Build history of the part. All positions in model axes, mm. A direction names the side the tool comes from. Round coordinates to 2 decimals unless told otherwise and drop trailing zeros. Write each loop counter-clockwise with the first axis right and the second up, starting at its lowest first coordinate (ties: lowest second). Pieces come first, ordered by that corner, then holes. Notation, with made-up numbers: M 3,-17 L 43,-17 A21 ccw 43,1 Z; hole C 35,88 d8. An arc over 180 degrees is marked long. Write item = value, one per line. Start each with the question number.
Q1. Probe L1, parallel to Z at x = 8, y = -5.5; L2, parallel to Z at x = 0.75, y = 1.5; L3, parallel to Y at x = -6, z = 11.5. List the from-to ranges inside material, lowest first.
Q2. Band-saw the part on A-A on y = 0. Write the cut outline in (x, z) (3 decimals), plus the area to 3 significant figures.
Q3. Band-saw the part on B-B on x = 0. Write the cut outline in (y, z) (3 decimals), plus the area to 3 significant figures.
Q4. Band-saw the part on C-C on z = 29. Write the cut outline in (x, y), plus the area to 3 significant figures.
Q5. Band-saw the part on D-D on y = 6. Write the cut outline in (x, z).
Q6. Pull direction Y, two halves, no side cores. Call faces 1 (the flat face through (0, -3.55, -1)), 2 (the flat face through (-6.037, 8.094, 3.414)), 3 (the flat face through (-1, 1, 26.7)): released by +Y, released by -Y, zero draft, split by the parting line, or undercut.
Q7. Tool access for faces 4 (the flat face through (0, 0, 34.4)), 5 (the cylindrical face through (0, -1, 30)), 6 (the flat face through (5.85, 8.24, 3.41)), 7 (the flat face through (0, 8, 5)), 8 (the flat face through (0, -5, 0)): list every direction of +Z, -Z, +X, -X, +Y, -Y with a clear straight run to the whole face (end or side of a thin tool).
Q8. Drop flat-ended pins along their axis: P1, Ø1, axis at x = 6, y = 8.5, coming from the +Z side; P2, Ø5, axis at x = 3, z = 13, coming from the +Y side; P3, Ø0.6, axis at x = 5, y = 8, coming from the -Z side. Give the stop position or say it passes through.
```python
from build123d import *

# Parameters (mm, degrees)
EXTRUDE_1_DEPTH = 25
SKETCH_3_R      = 1
EXTRUDE_2_DEPTH = 9.4
SKETCH_4_R      = 3.075
EXTRUDE_3_DEPTH = 1.7
EXTRUDE_4_DEPTH = 2.3
EXTRUDE_START   = 1.3
SKETCH_6_R      = 1
EXTRUDE_5_DEPTH = 1.3
SKETCH_8_W      = 8.5
SKETCH_8_H      = 5
EXTRUDE_6_DEPTH = 1.4
SKETCH_9_W      = 2
SKETCH_9_H      = 3.5
EXTRUDE_7_DEPTH = 0.1


with BuildPart() as part:
    # 草图2 → 凸台-拉伸1 (new body)
    with BuildSketch(Plane.XY):
        with BuildLine():
            Line((-6.557247898, -7.55), (6.557247898, -7.55))
            ThreePointArc((6.557247898, -7.55), (10, 0), (6.557247898, 7.55))
            Line((6.557247898, 7.55), (-6.557247898, 7.55))
            ThreePointArc((-6.557247898, 7.55), (-10, 0), (-6.557247898, -7.55))
        make_face()
    extrude(amount=EXTRUDE_1_DEPTH)

    # 草图3 → 凸台-拉伸2 (add)
    with BuildSketch(Plane.XY.offset(25)):
        Circle(SKETCH_3_R)
    extrude(amount=EXTRUDE_2_DEPTH)

    # 草图4 → 凸台-拉伸3 (add)
    with BuildSketch(Plane.XY.offset(25)):
        Circle(SKETCH_4_R)
    extrude(amount=EXTRUDE_3_DEPTH)

    # 草图5 → 凸台-拉伸4 (add)
    with BuildSketch(Plane(origin=(0, 0, 0), x_dir=(-1, 0, 0), z_dir=(0, 0, -1))):
        with BuildLine():
            Line((-3.521008378, -3.55), (3.521008378, -3.55))
            ThreePointArc((3.521008378, -3.55), (0, 5), (-3.521008378, -3.55))
        make_face()
    extrude(amount=EXTRUDE_4_DEPTH)

    # 草图6 → 凸台-拉伸5 (add)
    with BuildSketch(Plane(origin=(0, 0, -2.3), x_dir=(-1, 0, 0), z_dir=(0, 0, -1)).offset(EXTRUDE_START)):
        with Locations(Location((0, 0, 0), (0, 0, 180))):
            Circle(SKETCH_6_R)
    extrude(amount=-EXTRUDE_5_DEPTH)

    # 草图8 → 凸台-拉伸6 (add)
    with BuildSketch(Plane(origin=(0, 7.55, 0), x_dir=(1, 0, 0), z_dir=(0, 1, 0))):
        with Locations((0, -2.5)):
            Rectangle(SKETCH_8_W, SKETCH_8_H)
    extrude(amount=EXTRUDE_6_DEPTH)

    # 草图9 → 凸台-拉伸7 (add, symmetric)
    with BuildSketch(Plane(origin=(-1.929367668, 5.300894102, 0), x_dir=(0, 0, -1), z_dir=(-0.34202014332566943, 0.9396926207859081, 0))):
        with Locations((-3.4, -8.32594572)):
            Rectangle(SKETCH_9_W, SKETCH_9_H)
    extrude_7 = extrude(amount=EXTRUDE_7_DEPTH, both=True)

    # 镜向1: 凸台-拉伸7 across plane
    add(extrude_7.mirror(Plane(origin=(0, 0, 0), x_dir=(0, 0, 1), z_dir=(1, 0, 0))))


solid = part.part
```
Conclusion:
q1.L1 = 0 to 25
q1.L2 = -2.3 to 26.7
q1.L3 = -7.55 to 7.55
q2.outline = M -10,0 L -5,0 L -5,-2.3 L -1,-2.3 L -1,-3.6 L 1,-3.6 L 1,-2.3 L 5,-2.3 L 5,0 L 10,0 L 10,25 L 3.075,25 L 3.075,26.7 L 1,26.7 L 1,34.4 L -1,34.4 L -1,26.7 L -3.075,26.7 L -3.075,25 L -10,25 Z
q2.area = 551 mm^2
q3.outline = M -7.55,0 L -3.55,0 L -3.55,-2.3 L -1,-2.3 L -1,-3.6 L 1,-3.6 L 1,-2.3 L 5,-2.3 L 5,0 L 8.95,0 L 8.95,5 L 7.55,5 L 7.55,25 L 3.075,25 L 3.075,26.7 L 1,26.7 L 1,34.4 L -1,34.4 L -1,26.7 L -3.075,26.7 L -3.075,25 L -7.55,25 Z
q3.area = 433 mm^2
q4.outline = C 0,0 d2
q4.area = 3.14 mm^2
q5.outline = M -8,0 L 8,0 L 8,25 L -8,25 Z
q6.face_1 = released by -Y
q6.face_2 = undercut
q6.face_3 = zero draft
q7.face_4 = +Z, +X, -X, +Y, -Y
q7.face_5 = +Z
q7.face_6 = +Z, -Z, +Y
q7.face_7 = +Z, +X, -X, +Y
q7.face_8 = -Z
q8.P1 = 4.4
q8.P2 = 7.55
q8.P3 = 2.4
